Verification items for the finished model (mm, model axes). Face numbers are marked on the shaded views. A direction names the side the tool comes from. Coordinates: 2 decimals unless noted, no trailing zeros. Order: outer loops, then holes, each group sorted by start corner. A loop starts at its lowest first (then second) coordinate and runs counter-clockwise, first axis right, second up.
Q1. Cross-section at D-D, the plane y = -4.95. Record the boundary of the cut face in (x, z).
Q2. Thickness scan on line 1 (Y direction, x = 0, z = -1.3); line 2 (X direction, y = -3.5, z = 2.2); line 3 (Z direction, x = 2.5, y = -13). Record the ranges inside material, lowest first.
Q3. Depth check by flat-ended pin: P1, Ø1, axis at y = -6.5, z = -2, coming from the -X side; P2, Ø1.5, axis at y = 1, z = -0.5, coming from the -X side; P3, Ø4.5, axis at x = 8.57, y = -4.95, coming from the -Z side; P4, Ø1.5, axis at x = 0, z = -0.5, coming from the +Y side. Enter the tip coordinate at first touch or a pass-through.
Q4. Cross-section at C-C, the plane z = 0.65. Record the boundary of the cut face in (x, y).
Q5. Cross-section at A-A, the plane x = 0. Record the boundary of the cut face in (y, z) (3 decimals).
Q6. Draft check along Y on the marked faces 1, 2 and 3. Enter one of: pulls with the +Y half, pulls with the -Y half, needs draft (parallel to the pull), parting line crosses it, or undercut.
Q7. Set-up check for the marked faces 4, 5 and 6: record each of +Z, -Z, +X, -X, +Y, -Y from which the full face is reachable in a straight line by a thin tool's end or side.
Q8. Cross-section at B-B, the plane y = 0. Record the boundary of the cut face in (x, z) (3 decimals), and give its area (3 significant figures).
from build123d import *

# Parameters (mm, degrees)
SKETCH1_R           = 19.78095238
SKETCH1_R_2         = 1.8669
BOSS_EXTRUDE1_DEPTH = 2.794
SKETCH2_R           = 16.375
SKETCH2_R_2         = 4.5
CUT_EXTRUDE1_DEPTH  = 1.3
SKETCH3_R           = 3.6
CUT_EXTRUDE2_DEPTH  = 29.301220789


with BuildPart() as part:
    # Sketch1 → Boss-Extrude1 (new, symmetric)
    with BuildSketch(Plane.XY):
        Circle(SKETCH1_R)
        Circle(SKETCH1_R_2, mode=Mode.SUBTRACT)
    extrude(amount=BOSS_EXTRUDE1_DEPTH, both=True)

    # Sketch2 → Cut-Extrude1 (cut)
    with BuildSketch(Plane.XY.offset(2.794)):
        Circle(SKETCH2_R)
        Circle(SKETCH2_R_2, mode=Mode.SUBTRACT)
    cut_extrude1 = extrude(amount=-CUT_EXTRUDE1_DEPTH, mode=Mode.SUBTRACT)

    # Mirror1: Cut-Extrude1 across plane
    add(cut_extrude1.mirror(Plane.XY), mode=Mode.SUBTRACT)

    # Sketch3 → Cut-Extrude2 (cut, through all)
    with BuildSketch(Plane.XY.offset(1.494)):
        with Locations((0, 9.9)):
            Circle(SKETCH3_R)
        with Locations((8.573651497, -4.95)):
            Circle(SKETCH3_R)
        with Locations((-8.573651497, -4.95)):
            Circle(SKETCH3_R)
    extrude(amount=-CUT_EXTRUDE2_DEPTH, mode=Mode.SUBTRACT)


solid = part.part
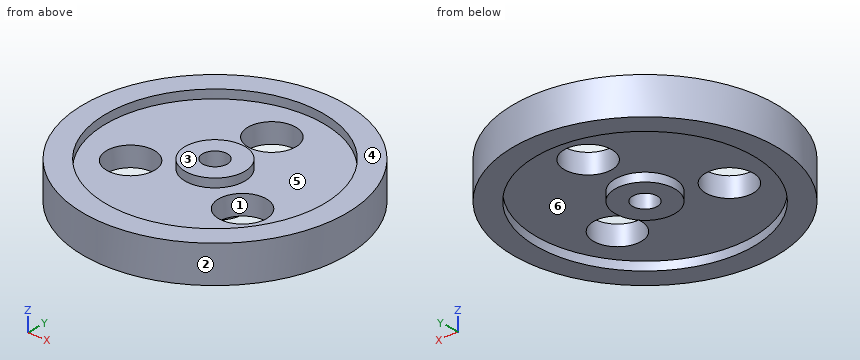
Check values:
1. outline: (-19.15, -2.79) - (-15.61, -2.79) - (-15.61, -1.49) - (-12.17, -1.49) - (-12.17, 1.49) - (-15.61, 1.49) - (-15.61, 2.79) - (-19.15, 2.79) - close; (-4.97, -1.49) - (4.97, -1.49) - (4.97, 1.49) - (-4.97, 1.49) - close; (12.17, -1.49) - (15.61, -1.49) - (15.61, -2.79) - (19.15, -2.79) - (19.15, 2.79) - (15.61, 2.79) - (15.61, 1.49) - (12.17, 1.49) - close
2. line 1: y = -19.78 to -1.87, 1.87 to 6.3, 13.5 to 19.78
2. line 2: x = -19.47 to -16, -2.83 to 2.83, 16 to 19.47
2. line 3: z = -1.49 to 1.49
3. P1: stops at x = -18.85
3. P2: stops at x = -19.78
3. P3: passes through
3. P4: stops at y = 19.78
4. outline: circle Ø39.56 at (0, 0); hole circle Ø7.2 at (-8.57, -4.95); hole circle Ø7.2 at (0, 9.9); hole circle Ø3.73 at (0, 0); hole circle Ø7.2 at (8.57, -4.95)
5. outline: (-19.781, -2.794) - (-16.375, -2.794) - (-16.375, -1.494) - (-4.5, -1.494) - (-4.5, -2.794) - (-1.867, -2.794) - (-1.867, 2.794) - (-4.5, 2.794) - (-4.5, 1.494) - (-16.375, 1.494) - (-16.375, 2.794) - (-19.781, 2.794) - close; (1.867, -2.794) - (4.5, -2.794) - (4.5, -1.494) - (6.3, -1.494) - (6.3, 1.494) - (4.5, 1.494) - (4.5, 2.794) - (1.867, 2.794) - close; (13.5, -1.494) - (16.375, -1.494) - (16.375, -2.794) - (19.781, -2.794) - (19.781, 2.794) - (16.375, 2.794) - (16.375, 1.494) - (13.5, 1.494) - close
6. face 1: undercut
6. face 2: parting line crosses it
6. face 3: needs draft
7. face 4: +Z, +X, -X, +Y, -Y
7. face 5: +Z
7. face 6: -Z
8. outline: (-19.781, -2.794) - (-16.375, -2.794) - (-16.375, -1.494) - (-4.5, -1.494) - (-4.5, -2.794) - (-1.867, -2.794) - (-1.867, 2.794) - (-4.5, 2.794) - (-4.5, 1.494) - (-16.375, 1.494) - (-16.375, 2.794) - (-19.781, 2.794) - close; (1.867, -2.794) - (4.5, -2.794) - (4.5, -1.494) - (16.375, -1.494) - (16.375, -2.794) - (19.781, -2.794) - (19.781, 2.794) - (16.375, 2.794) - (16.375, 1.494) - (4.5, 1.494) - (4.5, 2.794) - (1.867, 2.794) - close
8. area: 138 mm2
